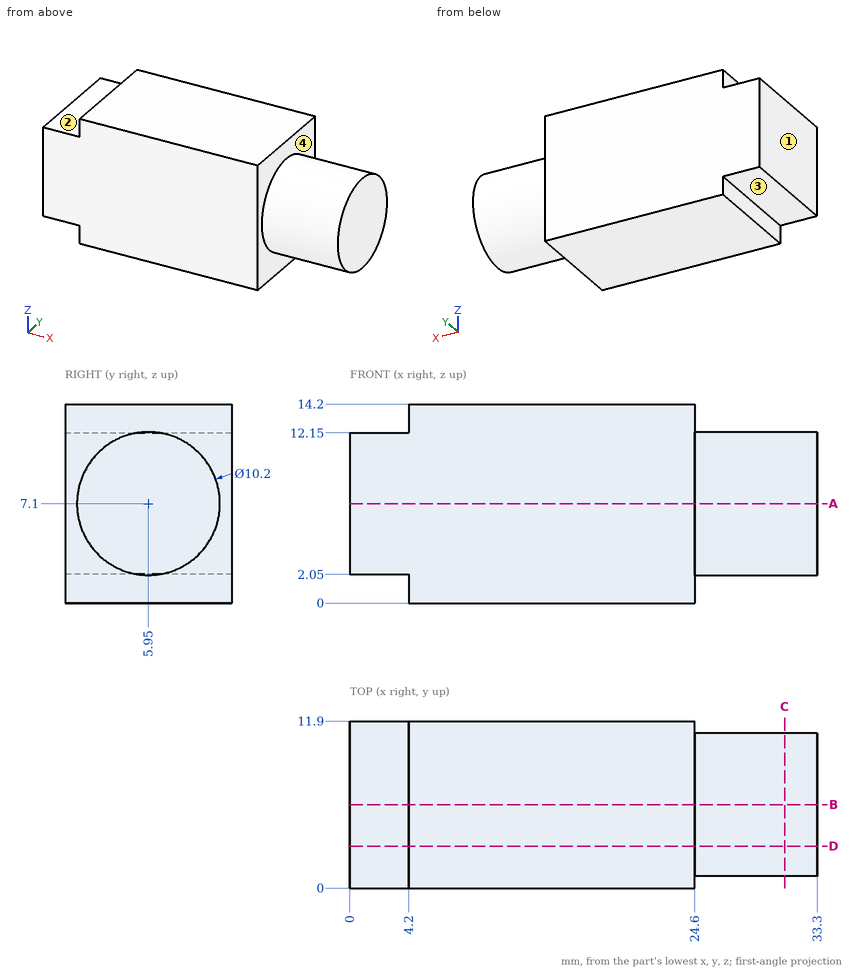
Geometry: see drawing. Coordinates: mm, zero at the bounding-box minimum. A direction names the side the tool comes from. Round coordinates to 2 decimals unless told otherwise and drop trailing zeros. Loops run counter-clockwise (first coordinate to the right, second up) from the corner with the lowest first, then second, coordinate; pieces in that order, holes last. Notation, with made-up numbers: M -13,26 L 41,26 A16 ccw 41,55 Z; hole C 13.25,37 d6. An arc over 180 degrees is marked long. Use a Markdown table: item, result. Add a question column.
1. Section query B-B on y = 5.95. Return the cut outline in (x, z).
2. Line query: line 1 (X direction, y = 10, z = 13.25); line 2 (X direction, y = 10, z = 3.5); line 3 (Y direction, x = 27, z = 8.25). Output: solid intervals per line, ascending.
3. Section query D-D on y = 3. Return the cut outline in (x, z).
4. Reachability of the marked faces 1, 2, 3 and 4 from +Z, -Z, +X, -X, +Y, -Y: full face, straight path, thin tool, end or side. Return the list, or none.
5. Section query A-A on z = 7.1. Return the cut outline in (x, y).
6. Contact query for flat-ended pins moving along their axis: P1, Ø4, axis at x = 15, z = 11.5, coming from the -Y side; P2, Ø2, axis at x = 2, y = 8, coming from the +Z side; P3, Ø4.5, axis at x = 1.5, y = 3, coming from the -Z side; P4, Ø1.6, axis at y = 6, z = 13.5, coming from the -X side. Output: stop coordinate, or through.
7. Section query C-C on x = 31. Return the cut outline in (y, z), then the cut area to 3 significant figures.
Reported:
| question | item | result |
|---|---|---|
| 1 | outline | M 0,2.05 L 4.2,2.05 L 4.2,0 L 24.6,0 L 24.6,2 L 33.3,2 L 33.3,12.2 L 24.6,12.2 L 24.6,14.2 L 4.2,14.2 L 4.2,12.15 L 0,12.15 Z |
| 2 | line 1 | x = 4.2 to 24.6 |
| 2 | line 2 | x = 0 to 24.6 |
| 2 | line 3 | y = 0.98 to 10.92 |
| 3 | outline | M 0,2.05 L 4.2,2.05 L 4.2,0 L 24.6,0 L 24.6,2.94 L 33.3,2.94 L 33.3,11.26 L 24.6,11.26 L 24.6,14.2 L 4.2,14.2 L 4.2,12.15 L 0,12.15 Z |
| 4 | face 1 | +Z, -Z, -X, +Y, -Y |
| 4 | face 2 | +Z, -X, +Y, -Y |
| 4 | face 3 | -Z, -X, +Y, -Y |
| 4 | face 4 | +X |
| 5 | outline | M 0,0 L 24.6,0 L 24.6,0.85 L 33.3,0.85 L 33.3,11.05 L 24.6,11.05 L 24.6,11.9 L 0,11.9 Z |
| 6 | P1 | stops at y = 0 |
| 6 | P2 | stops at z = 12.15 |
| 6 | P3 | stops at z = 2.05 |
| 6 | P4 | stops at x = 4.2 |
| 7 | outline | C 5.95,7.1 d10.2 |
| 7 | area | 81.7 mm² |
